Geometry: final body of the model. Coordinates: model frame, mm. A direction names the side the tool comes from. Give positions to 0.01 mm unless a question says otherwise; leave off trailing zeros. Write each loop counter-clockwise with the first axis right and the second up, starting at its lowest first coordinate (ties: lowest second). Pieces come first, ordered by that corner, then holes.
from build123d import *

# Parameters (mm, degrees)
F1_DEPTH = 101.6


with BuildPart() as f1:
    # F0 (on Front) → F1 (new body)
    with BuildSketch(Plane.XZ):
        with BuildLine():
            Line((0, -50.8), (0, -46.5666666667))
            ThreePointArc((0, -46.5666666667), (-39.1654835814, -34.5533971745), (-64.859084298, -2.6458333333))
            Line((-64.859084298, -2.6458333333), (-69.0924176313, -2.6458333333))
            Line((-69.0924176313, -2.6458333333), (-69.0924176313, 0))
            Line((-69.0924176313, 0), (-101.6, 0))
            Line((-101.6, 0), (-101.6, -50.8))
            Line((-101.6, -50.8), (0, -50.8))
        make_face()
    extrude(amount=F1_DEPTH)


solid = f1.part
Q1. Ray query, line 1 along X through (y, z) = (-77, -2.5); line 2 along X through (y, z) = (-97, -16); line 3 along Z through (x, y) = (-38, -30). Return the intervals inside material, ascending.
Filled sheet:
line 1: x = -101.6 to -69.09
line 2: x = -101.6 to -57.76
line 3: z = -50.8 to -35.33
Q2. Section A-A on y = -25.5. Output: boundary loops of the cut face in (x, z).
Filled sheet:
outline: (-101.6, -50.8) - (0, -50.8) - (0, -46.57) arc R69.85 cw to (-64.86, -2.65) - (-69.09, -2.65) - (-69.09, 0) - (-101.6, 0) - close
Q3. Pin query (flat end, axial travel): P1, Ø5, axis at y = -52, z = -18, coming from the +X side; P2, Ø3, axis at y = -27, z = -1, coming from the +X side; P3, Ø4, axis at x = -64, y = -89, coming from the +Z side. Return the tip coordinate at first contact, or that it passes through.
Filled sheet:
P1: stops at x = -54.42
P2: stops at x = -69.09
P3: stops at z = -2.65
Q4. Access query for faces 1 (the flat face through (-69.092, -50, -1)), 2 (the flat face through (-74, -101.6, -31)). Directions: +Z, -Z, +X, -X, +Y, -Y. A direction counts if a zero-diameter tool reaches every point of the face in a straight line with its end or side. Return the directions, or none.
Filled sheet:
face 1: +Z, +X, +Y, -Y
face 2: +Z, -Z, +X, -X, -Y
Q5. Section C-C on x = -50.5. Output: boundary loops of the cut face in (y, z).
Filled sheet:
outline: (-101.6, -50.8) - (0, -50.8) - (0, -24.97) - (-101.6, -24.97) - close
Q6. Section B-B on z = -30. Output: boundary loops of the cut face in (x, y).
Filled sheet:
outline: (-101.6, -101.6) - (-45.17, -101.6) - (-45.17, 0) - (-101.6, 0) - close
